from build123d import *

# Parameters (mm, degrees)
SKETCH_1_W          = 6
SKETCH_1_H          = 6
EXTRUDE_1_DEPTH     = 40
SKETCH_2_R          = 1.6
CUT_EXTRUDE_1_DEPTH = 40
SKETCH_3_R          = 1.6
CUT_EXTRUDE_2_DEPTH = 40
FILLET_1_R          = 0.1


with BuildPart() as part:
    # 草图1 → 凸台-拉伸1 (new body)
    with BuildSketch(Plane.XY):
        Rectangle(SKETCH_1_W, SKETCH_1_H)
    extrude(amount=EXTRUDE_1_DEPTH)

    # 草图2 → 切除-拉伸1 (cut)
    with BuildSketch(Plane.ZY.offset(3)):
        with Locations(Location((15, 0, 0), (0, 0, 270))):
            Circle(SKETCH_2_R)
        with Locations(Location((35, 0, 0), (0, 0, 270))):
            Circle(SKETCH_2_R)
    extrude(amount=-CUT_EXTRUDE_1_DEPTH, mode=Mode.SUBTRACT)

    # 草图3 → 切除-拉伸2 (cut)
    with BuildSketch(Plane(origin=(0, 3, 0), x_dir=(1, 0, 0), z_dir=(0, 1, 0))):
        with Locations(Location((0, -5, 0), (0, 0, 270))):
            Circle(SKETCH_3_R)
        with Locations(Location((0, -25, 0), (0, 0, 270))):
            Circle(SKETCH_3_R)
    extrude(amount=-CUT_EXTRUDE_2_DEPTH, mode=Mode.SUBTRACT)

    # 圆角1
    fillet_1_edges = [part.edges().sort_by_distance(p)[0] for p in [
        (-3, 0, 40),
        (0, -3, 40),
        (3, 0, 40),
        (0, -3, 0),
        (-3, 0, 0),
        (0, 3, 0),
        (3, 0, 0),
        (3, -3, 20),
        (-3, -3, 20),
        (-3, 3, 20),
        (3, 3, 20),
        (0, 3, 40),
    ]]
    fillet(fillet_1_edges, radius=FILLET_1_R)


solid = part.part
Check sheet for the modelled part. Datum: model origin and axes. Units: mm. Round coordinates to 2 decimals unless told otherwise and drop trailing zeros. Loops run counter-clockwise (first coordinate to the right, second up) from the corner with the lowest first, then second, coordinate; pieces in that order, holes last. Notation, with made-up numbers: (-17.5, 79) -> (40.5, 79) arc R33 cw to (40.5, 117) -> close; hole circle Ø11 at (-15.75, -38). An arc over 180 degrees is marked (long way). Put each result on its own line as item: value. Start each with the question number.
1. Scan lines: probe 1 along Z at (x, y) = (-1.7, 0); probe 2 along Z at (x, y) = (-0.3, -0.6); probe 3 along Z at (x, y) = (-0.95, 0.95). Record each from-to range of solid material in increasing order.
2. Section check D-D (x = 2.45). Enter the section's corners in (y, z), plus the area to 3 significant figures.
3. Section check A-A (x = 0). Enter the section's corners in (y, z), plus the area to 3 significant figures.
4. Draft check along Z on faces 1 (the face through (-0.04, -0.74, 33.58)), 2 (the face through (0, 0, 0)), 3 (the face through (0, -3, 20)), 4 (the face through (-0.042, 0.208, 16.586)). Enter one of: +Z half, -Z half, draft (parallel to the pull), parting line (faces both ways), or undercut.
5. Gauge pin test, flat end, axial feed: pin 1 (3 mm diameter, centred on x = 0.5, z = 24.5, fed in from +Y). Record the tip position at first contact, or that the pin passes through.
6. Section check B-B (y = -0.5). Enter the section's corners in (x, z).
7. Section check C-C (z = 35). Enter the section's corners in (x, y).
Findings:
1. probe 1: z = 0 to 13.4, 16.6 to 33.4, 36.6 to 40
1. probe 2: z = 0 to 3.43, 6.57 to 13.52, 16.48 to 23.43, 26.57 to 33.52, 36.48 to 40
1. probe 3: z = 0 to 3.71, 6.29 to 13.71, 16.29 to 23.71, 26.29 to 33.71, 36.29 to 40
2. outline: (-3, 0.1) arc R0.1 ccw to (-2.9, 0) -> (2.9, 0) arc R0.1 ccw to (3, 0.1) -> (3, 39.9) arc R0.1 ccw to (2.9, 40) -> (-2.9, 40) arc R0.1 ccw to (-3, 39.9) -> close; hole circle Ø3.2 at (0, 15); hole circle Ø3.2 at (0, 35)
2. area: 224 mm^2
3. outline: (-3, 0.1) arc R0.1 ccw to (-2.9, 0) -> (2.9, 0) arc R0.1 ccw to (3, 0.1) -> (3, 3.4) -> (-3, 3.4) -> close; (-3, 6.6) -> (3, 6.6) -> (3, 23.4) -> (-3, 23.4) -> close; (-3, 26.6) -> (3, 26.6) -> (3, 39.9) arc R0.1 ccw to (2.9, 40) -> (-2.9, 40) arc R0.1 ccw to (-3, 39.9) -> close; hole circle Ø3.2 at (0, 15); hole circle Ø3.2 at (0, 35)
3. area: 186 mm^2
4. face 1: undercut
4. face 2: -Z half
4. face 3: draft
4. face 4: undercut
5. pin 1: stops at y = 3
6. outline: (-3, 0.1) arc R0.1 ccw to (-2.9, 0) -> (2.9, 0) arc R0.1 ccw to (3, 0.1) -> (3, 13.48) -> (-3, 13.48) -> close; (-3, 16.52) -> (3, 16.52) -> (3, 33.48) -> (-3, 33.48) -> close; (-3, 36.52) -> (3, 36.52) -> (3, 39.9) arc R0.1 ccw to (2.9, 40) -> (-2.9, 40) arc R0.1 ccw to (-3, 39.9) -> close; hole circle Ø3.2 at (0, 5); hole circle Ø3.2 at (0, 25)
7. outline: (-3, -2.9) arc R0.1 ccw to (-2.9, -3) -> (2.9, -3) arc R0.1 ccw to (3, -2.9) -> (3, -1.6) -> (-3, -1.6) -> close; (-3, 1.6) -> (3, 1.6) -> (3, 2.9) arc R0.1 ccw to (2.9, 3) -> (-2.9, 3) arc R0.1 ccw to (-3, 2.9) -> close
